```python
from build123d import *

# Parameters (mm, degrees)
SKETCH1_R           = 14.2875
SKETCH1_R_2         = 3.2639
SKETCH1_R_3         = 2.4892
SKETCH1_R_4         = 12.7
BOSS_EXTRUDE1_DEPTH = 6.35
FILLET1_R           = 12.7
CUT_EXTRUDE1_DEPTH  = 1111.646166548
FILLET2_R           = 3.175


with BuildPart() as part:
    # Sketch1 → Boss-Extrude1 (new body)
    with BuildSketch(Plane(origin=(0, 0, 0), x_dir=(0, 0, -1), z_dir=(1, 0, 0))):
        with BuildLine():
            ThreePointArc((-970.159977951, 486.471044057), (-972.554742028, 481.307456029), (-969.849900837, 476.299325595))
            Line((-969.849900837, 476.299325595), (-957.32612323, 467.530082108))
            ThreePointArc((-957.32612323, 467.530082108), (-952.814366358, 447.526291127), (-933.279921362, 441.288257591))
            Line((-933.279921362, 441.288257591), (-904.317406585, 391.123710482))
            ThreePointArc((-904.317406585, 391.123710482), (-899.31875, 359.420584766), (-869.363709458, 370.943184037))
            Line((-869.363709458, 370.943184037), (-793.75, 370.943184037))
            ThreePointArc((-793.75, 370.943184037), (-788.345816721, 373.958922036), (-788.074736079, 380.141671253))
            Line((-788.074736079, 380.141671253), (-821.515081147, 446.767486803))
            ThreePointArc((-821.515081147, 446.767486803), (-816.600560548, 454.425027508), (-815.456796251, 463.451779173))
            Line((-815.456796251, 463.451779173), (-790.191295152, 474.402994585))
            ThreePointArc((-790.191295152, 474.402994585), (-754.524902303, 483.694296655), (-783.206575716, 506.841250736))
            Line((-783.206575716, 506.841250736), (-808.094430848, 534.22843431))
            ThreePointArc((-808.094430848, 534.22843431), (-810.224397121, 535.764782193), (-812.79386882, 536.307862598))
            Line((-812.79386882, 536.307862598), (-848.714893304, 536.307862598))
            ThreePointArc((-848.714893304, 536.307862598), (-850.783311047, 535.961540474), (-852.626110261, 534.96035017))
            Line((-852.626110261, 534.96035017), (-873.884548632, 518.339346434))
            ThreePointArc((-873.884548632, 518.339346434), (-875.222451174, 517.536616274), (-876.715710426, 517.084360008))
            Line((-876.715710426, 517.084360008), (-945.294856051, 505.247433425))
            ThreePointArc((-945.294856051, 505.247433425), (-946.812001144, 504.784530233), (-948.167088373, 503.960062407))
            Line((-948.167088373, 503.960062407), (-970.159977951, 486.471044057))
        make_face()
        with Locations((-774.7, 488.038469669)):
            Circle(SKETCH1_R, mode=Mode.SUBTRACT)
        with Locations((-835.998805319, 461.468784037)):
            Circle(SKETCH1_R, mode=Mode.SUBTRACT)
        with Locations((-889, 377.293184037)):
            Circle(SKETCH1_R, mode=Mode.SUBTRACT)
        with Locations((-937.598805319, 461.468784037)):
            Circle(SKETCH1_R, mode=Mode.SUBTRACT)
        with Locations((-850.9, 377.293184037)):
            Circle(SKETCH1_R_2, mode=Mode.SUBTRACT)
        with Locations((-831.85, 377.293184037)):
            Circle(SKETCH1_R_2, mode=Mode.SUBTRACT)
        with Locations((-812.8, 377.293184037)):
            Circle(SKETCH1_R_2, mode=Mode.SUBTRACT)
        with Locations((-793.75, 377.293184037)):
            Circle(SKETCH1_R_2, mode=Mode.SUBTRACT)
        with Locations((-966.207690466, 481.500941076)):
            Circle(SKETCH1_R_2, mode=Mode.SUBTRACT)
        with Locations((-944.214800888, 498.989959427)):
            Circle(SKETCH1_R_2, mode=Mode.SUBTRACT)
        with Locations((-868.854381062, 511.997350355)):
            Circle(SKETCH1_R_2, mode=Mode.SUBTRACT)
        with Locations((-848.714893304, 494.036838113)):
            Circle(SKETCH1_R_3, mode=Mode.SUBTRACT)
        with Locations((-812.79386882, 494.036838113)):
            Circle(SKETCH1_R_3, mode=Mode.SUBTRACT)
        with Locations((-830.754381062, 511.997350355)):
            Circle(SKETCH1_R_4, mode=Mode.SUBTRACT)
        with Locations((-848.714893304, 529.957862598)):
            Circle(SKETCH1_R_3, mode=Mode.SUBTRACT)
        with Locations((-812.79386882, 529.957862598)):
            Circle(SKETCH1_R_3, mode=Mode.SUBTRACT)
    extrude(amount=BOSS_EXTRUDE1_DEPTH)

    # Fillet1
    fillet1_edges = [part.edges().sort_by_distance(p)[0] for p in [
        (3.175, 391.123710482, 904.317406585),
        (3.175, 441.288257591, 933.279921362),
        (3.175, 467.530082108, 957.32612323),
        (3.175, 506.841250736, 783.206575716),
        (3.175, 474.402994585, 790.191295152),
        (3.175, 463.451779173, 815.456796251),
        (3.175, 446.767486803, 821.515081147),
        (3.175, 370.943184037, 869.363709458),
    ]]
    fillet(fillet1_edges, radius=FILLET1_R)

    # Sketch2 → Cut-Extrude1 (cut, through all)
    with BuildSketch(Plane(origin=(6.35, 0, 0), x_dir=(0, 0, -1), z_dir=(1, 0, 0))):
        with BuildLine():
            Line((-941.533962306, 493.008784522), (-955.598677388, 481.824348785))
            Line((-955.598677388, 481.824348785), (-950.041702488, 477.93331307))
            ThreePointArc((-950.041702488, 477.93331307), (-937.835924045, 482.10492178), (-925.537513496, 478.214877486))
            Line((-925.537513496, 478.214877486), (-894.3242024, 501.157303389))
            Line((-894.3242024, 501.157303389), (-941.533962306, 493.008784522))
        make_face()
        with BuildLine():
            Line((-852.026643719, 474.469353351), (-870.512088457, 502.898105526))
            Line((-870.512088457, 502.898105526), (-910.437563384, 473.552059946))
            ThreePointArc((-910.437563384, 473.552059946), (-911.574059703, 470.004314737), (-908.557177951, 467.818784037))
            Line((-908.557177951, 467.818784037), (-855.635095861, 467.818784037))
            ThreePointArc((-855.635095861, 467.818784037), (-854.138266208, 471.310855207), (-852.026643719, 474.469353351))
        make_face()
        with BuildLine():
            ThreePointArc((-917.962514777, 455.118784037), (-919.726206049, 451.150034037), (-922.281398734, 447.638257591))
            Line((-922.281398734, 447.638257591), (-893.318883957, 397.473710482))
            ThreePointArc((-893.318883957, 397.473710482), (-888.604427978, 397.926892599), (-883.91080583, 397.29334676))
            Line((-883.91080583, 397.29334676), (-851.835056229, 448.235509183))
            ThreePointArc((-851.835056229, 448.235509183), (-854.065907119, 451.494505176), (-855.635095861, 455.118784037))
            Line((-855.635095861, 455.118784037), (-917.962514777, 455.118784037))
        make_face()
        with BuildLine():
            Line((-804.042101766, 383.643184037), (-832.86560899, 441.07051237))
            ThreePointArc((-832.86560899, 441.07051237), (-836.996855705, 440.855431527), (-841.08799949, 441.468621314))
            Line((-841.08799949, 441.468621314), (-873.16374909, 390.526458891))
            ThreePointArc((-873.16374909, 390.526458891), (-870.9328982, 387.267462898), (-869.363709458, 383.643184037))
            Line((-869.363709458, 383.643184037), (-804.042101766, 383.643184037))
        make_face()
    extrude(amount=-CUT_EXTRUDE1_DEPTH, mode=Mode.SUBTRACT)

    # Fillet2
    fillet2_edges = [part.edges().sort_by_distance(p)[0] for p in [
        (3.175, 478.214877486, 925.537513496),
        (3.175, 477.93331307, 950.041702488),
        (3.175, 481.824348785, 955.598677388),
        (3.175, 493.008784522, 941.533962306),
        (3.175, 501.157303389, 894.3242024),
        (3.175, 397.29334676, 883.91080583),
        (3.175, 397.473710482, 893.318883957),
        (3.175, 447.638257591, 922.281398734),
        (3.175, 455.118784037, 917.962514777),
        (3.175, 455.118784037, 855.635095861),
        (3.175, 448.235509183, 851.835056229),
        (3.175, 383.643184037, 869.363709458),
        (3.175, 390.526458891, 873.16374909),
        (3.175, 441.468621314, 841.08799949),
        (3.175, 441.07051237, 832.86560899),
        (3.175, 383.643184037, 804.042101766),
        (3.175, 502.898105526, 870.512088457),
        (3.175, 474.469353351, 852.026643719),
        (3.175, 467.818784037, 855.635095861),
    ]]
    fillet(fillet2_edges, radius=FILLET2_R)


solid = part.part
```
Here's how the part is built. I have some questions about the finished solid (model axes, mm). A direction names the side the tool comes from. Round coordinates to 2 decimals unless told otherwise and drop trailing zeros. Order: outer loops, then holes, each group sorted by start corner. A loop starts at its lowest first (then second) coordinate and runs counter-clockwise, first axis right, second up. Notation, with made-up numbers: M -32.5,67.5 L -9.5,67.5 A21 cw -9.5,102.5 Z; hole C 28,1 d5. An arc over 180 degrees is marked long. Answer as CSV lines item,"result".
Item 1: Imagine slicing it at C-C on x = 1. Give the number of separate pieces and of enclosed holes in the cut face, and give its area (3 significant figures).
From the geometry:
separate pieces,"1"
enclosed holes,"20"
area,"12,600 mm2"
Item 2: Imagine slicing it at B-B on z = 889. List the corners of the cut face in (x, y) for me, and give its area (3 significant figures).
From the geometry:
outline,"M 0,356.66 L 6.35,356.66 L 6.35,363.01 L 0,363.01 Z; M 0,391.58 L 6.35,391.58 L 6.35,397.93 L 0,397.93 Z; M 0,455.12 L 6.35,455.12 L 6.35,467.82 L 0,467.82 Z; M 0,489.31 L 6.35,489.31 L 6.35,514.96 L 0,514.96 Z"
area,"324 mm2"
Item 3: Please list where these lines run through material, in increasing order: L1, parallel to Z at x = 5.75, y = 433.5; L2, parallel to Z at x = 4.75, y = 418.5; L3, parallel to Z at x = 5, y = 375. Write a range as [from, to].
From the geometry:
L1,"[814.86, 829.07], [846.11, 861.11], [914.12, 928.78]"
L2,"[807.33, 821.54], [855.55, 870.56], [905.46, 920.12]"
L3,"[787.83, 791.43], [796.07, 810.48], [815.12, 829.53], [834.17, 848.58], [853.22, 874.9], [903.1, 909.51]"
Item 4: We'd pull the mould along Y, two halves only. Please class faces 1 (the flat face through (3.131, 474.16, 966.794)), 2 (the cylindrical face through (3.131, 501.465, 870.736)), 3 (the flat face through (3.131, 526.766, 863.107)), 4 (the cylindrical face through (3.131, 483.156, 754.648)): +Y half, -Y half, draft (parallel to the pull), parting line (faces both ways), or undercut.
From the geometry:
face 1,"-Y half"
face 2,"undercut"
face 3,"+Y half"
face 4,"parting line"
Item 5: Imagine slicing it at A-A on z = 774.7. List the corners of the cut face in (x, y) for me, and give its area (3 significant figures).
From the geometry:
outline,"M 0,467.4 L 6.35,467.4 L 6.35,473.75 L 0,473.75 Z; M 0,502.33 L 6.35,502.33 L 6.35,508.68 L 0,508.68 Z"
area,"80.6 mm2"
Item 6: For pin 1 (1.9 mm diameter, centred on x = 2.5, z = 890, fed in from +Y); pin 2 (1.5 mm diameter, centred on x = 2, y = 406.5, fed in from -Z); pin 3 (1 mm diameter, centred on x = 1.5, z = 798.5, fed in from +Y); pin 4 (8 mm diameter, centred on y = 515.5, z = 804.5, fed in from -X), each with a flat end and sliding along its axis, tell me the tip position at first contact or that it passes through.
From the geometry:
pin 1,"y = 514.96"
pin 2,"z = 800.93"
pin 3,"y = 524.22"
pin 4,"x = 0"
Item 7: Which directions (+Z, -Z, +X, -X, +Y, -Y) give clear straight access to the entire face, cutting with the end or side of a thin tool? Please do faces 5 (the cylindrical face through (3.131, 454.385, 816.615)), 6 (the cylindrical face through (3.13, 535.75, 810.19)), 7 (the flat face through (3.219, 496.047, 923.934)).
From the geometry:
face 5,"-Z, +X, -X"
face 6,"-Z, +X, -X, +Y"
face 7,"+X, -X"
